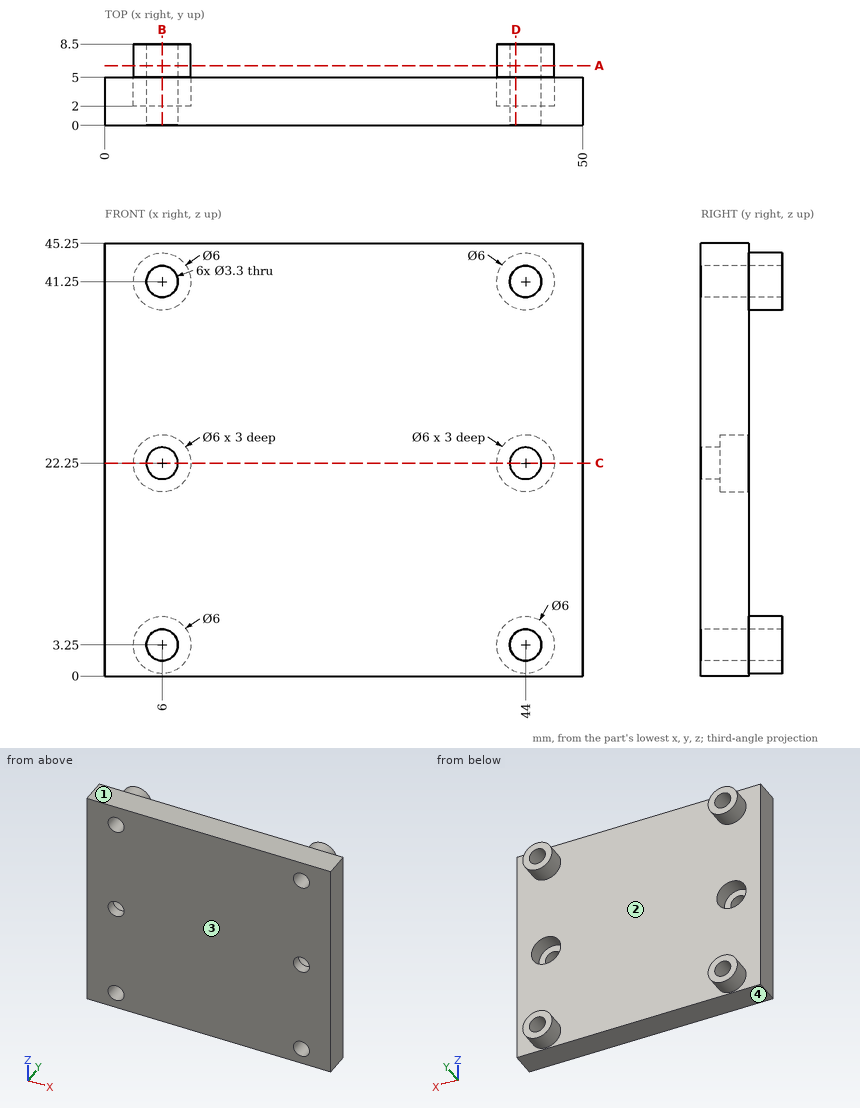
Drawing for the job (mm, zero at the part's lowest x, y, z). Round coordinates to 2 decimals unless told otherwise and drop trailing zeros. Loops run counter-clockwise (first coordinate to the right, second up) from the corner with the lowest first, then second, coordinate; pieces in that order, holes last. Notation, with made-up numbers: (-14.75, 21) - (16.25, 21) arc R33 cw to (16.25, 59) - close; hole circle Ø4 at (45.5, 61). An arc over 180 degrees is marked (long way). Return JSON: item names as keys, results as strings. Group by question number.
Q1. Band-saw the part on B-B on x = 6. Give the cut face in (y, z).
Q2. Band-saw the part on C-C on z = 22.25. Give the cut face in (x, y).
Q3. Drill centre lines: line 1 along X through (y, z) = (3.25, 3.25); line 2 along Z through (x, y) = (6, 1.15); line 3 along Z through (x, y) = (44, 4.75). Where is each one in solid material? Low to high. Write a range as [from, to].
Q4. Band-saw the part on D-D on x = 43. Give the cut face in (y, z), plus the area to 3 significant figures.
Q5. Two-plate mould, pull along Z, no slides. Class the marked faces 1, 2, 3 and 4: +Z half, -Z half, draft (parallel to the pull), parting line (faces both ways), or undercut.
Q6. Flat gauge pins, fed straight in: pin 1 Ø7 at (x, z) = (6, 22.25) entering from +Y; pin 2 Ø3.5 at (x, z) = (44, 22.25) entering from +Y. Where does each tip first touch, or does it go through?
Q7. Band-saw the part on A-A on y = 6.25. Give the cut face in (x, z).
Solutions:
{
 "1": {"outline": "(0, 0) - (5, 0) - (5, 0.25) - (8.5, 0.25) - (8.5, 1.6) - (0, 1.6) - close; (0, 4.9) - (8.5, 4.9) - (8.5, 6.25) - (5, 6.25) - (5, 19.25) - (2, 19.25) - (2, 20.6) - (0, 20.6) - close; (0, 23.9) - (2, 23.9) - (2, 25.25) - (5, 25.25) - (5, 38.25) - (8.5, 38.25) - (8.5, 39.6) - (0, 39.6) - close; (0, 42.9) - (8.5, 42.9) - (8.5, 44.25) - (5, 44.25) - (5, 45.25) - (0, 45.25) - close"},
 "2": {"outline": "(0, 0) - (4.35, 0) - (4.35, 2) - (3, 2) - (3, 5) - (0, 5) - close; (7.65, 0) - (42.35, 0) - (42.35, 2) - (41, 2) - (41, 5) - (9, 5) - (9, 2) - (7.65, 2) - close; (45.65, 0) - (50, 0) - (50, 5) - (47, 5) - (47, 2) - (45.65, 2) - close"},
 "3": {"line 1": "x = [0, 4.35], [7.65, 42.35], [45.65, 50]", "line 2": "z = [0, 1.6], [4.9, 20.6], [23.9, 39.6], [42.9, 45.25]", "line 3": "z = [0, 1.6], [4.9, 19.25], [25.25, 39.6], [42.9, 45.25]"},
 "4": {"outline": "(0, 0) - (5, 0) - (5, 0.42) - (8.5, 0.42) - (8.5, 1.94) - (0, 1.94) - close; (0, 4.56) - (8.5, 4.56) - (8.5, 6.08) - (5, 6.08) - (5, 19.42) - (2, 19.42) - (2, 20.94) - (0, 20.94) - close; (0, 23.56) - (2, 23.56) - (2, 25.08) - (5, 25.08) - (5, 38.42) - (8.5, 38.42) - (8.5, 39.94) - (0, 39.94) - close; (0, 42.56) - (8.5, 42.56) - (8.5, 44.08) - (5, 44.08) - (5, 45.25) - (0, 45.25) - close", "area": "199 mm^2"},
 "5": {"face 1": "+Z half", "face 2": "undercut", "face 3": "draft", "face 4": "-Z half"},
 "6": {"pin 1": "stops at y = 5", "pin 2": "stops at y = 2"},
 "7": {"outline": "circle Ø6 at (6, 3.25); circle Ø6 at (6, 41.25); circle Ø6 at (44, 3.25); circle Ø6 at (44, 41.25); hole circle Ø3.3 at (6, 3.25); hole circle Ø3.3 at (6, 41.25); hole circle Ø3.3 at (44, 3.25); hole circle Ø3.3 at (44, 41.25)"}
}
